The listing builds one solid part. Answer for the finished solid, in the listing's coordinates (mm). A direction names the side the tool comes from. Give positions to 0.01 mm unless a question says otherwise; leave off trailing zeros. Order: outer loops, then holes, each group sorted by start corner. A loop starts at its lowest first (then second) coordinate and runs counter-clockwise, first axis right, second up. Notation, with made-up numbers: (-39.5, 27) - (4.5, 27) arc R14 ccw to (4.5, 43) - close; hole circle Ø11 at (56, 70.25). An arc over 180 degrees is marked (long way). Answer as CSV lines item,"result". Start each with the question number.
1. Flat-ended cylindrical pins translate along their axes: pin 1 (8 mm diameter, centred on x = 14.5, z = -11.5, fed in from -Y); pin 2 (15 mm diameter, centred on x = 9.5, z = -4.5, fed in from -Y); pin 3 (1 mm diameter, centred on y = 0.5, z = 1, fed in from +X). Find the tip coordinate at first contact, or state that the pin passes through.
2. Which of the six approach directions +Z, -Z, +X, -X, +Y, -Y give full straight-line access (tool end or side, diameter ignored) to faces 4 (the cylindrical face through (12.285, 0.986, 9.699)), 5 (the cylindrical face through (-19.976, -0.246, -11.783)), 6 (the flat face through (22, 1, 13))?
3. Consider line 1 along X through (y, z) = (1.5, -10); line 2 along Z through (x, y) = (20, 0.95); line 3 along X through (y, z) = (1.2, 0.25). Determine where each line is inside the solid, lowest interval first. Write a range as [from, to].
4. Determine the mould class of faces 1 (the flat face through (0, 1, 15)), 2 (the flat face through (10, -2.4, -3)), 3 (the flat face through (17, 1, -5)) for opening direction Z: +Z half, -Z half, draft (parallel to the pull), parting line (faces both ways), or undercut.
5. Section C-C on y = 1.05 is taken. Give the vertices of the cut face in (x, z), and give its area (3 significant figures).
6. Section D-D on z = -10 is taken. Give the vertices of the cut face in (x, y).
7. Section B-B on z = 8.5 is taken. Give the vertices of the cut face in (x, y), and give its area (3 significant figures).
8. Section A-A on x = 17 is taken. Give the vertices of the cut face in (y, z), and give its area (3 significant figures).
from build123d import *

# Parameters (mm, degrees)
SKETCH1_W           = 44
SKETCH1_H           = 30
SKETCH1_R           = 1.2192
SKETCH1_R_2         = 1.55
BOSS_EXTRUDE1_DEPTH = 2
SKETCH2_R           = 1
BOSS_EXTRUDE2_DEPTH = 1.5
FILLET1_R           = 1
SKETCH4_R           = 1
BOSS_EXTRUDE3_DEPTH = 2.4
SKETCH5_W           = 10
SKETCH5_H           = 15
CUT_EXTRUDE1_DEPTH  = 27.988145546
FILLET2_R           = 1


with BuildPart() as part:
    # Sketch1 → Boss-Extrude1 (new body)
    with BuildSketch(Plane(origin=(0, 0, 0), x_dir=(1, 0, 0), z_dir=(0, 1, 0))):
        Rectangle(SKETCH1_W, SKETCH1_H)
        with Locations(Location((17, 10, 0), (0, 0, 270))):
            Circle(SKETCH1_R, mode=Mode.SUBTRACT)
        with Locations(Location((-6, 10, 0), (0, 0, 270))):
            Circle(SKETCH1_R_2, mode=Mode.SUBTRACT)
    extrude(amount=BOSS_EXTRUDE1_DEPTH)

    # Sketch2 → Boss-Extrude2 (add)
    with BuildSketch(Plane(origin=(0, 0, 0), x_dir=(-1, 0, 0), z_dir=(0, -1, 0))):
        with Locations(Location((19, 12, 0), (0, 0, 90))):
            Circle(SKETCH2_R)
        with Locations(Location((-10, -12.5, 0), (0, 0, 90))):
            Circle(SKETCH2_R)
    extrude(amount=BOSS_EXTRUDE2_DEPTH)

    # Fillet1
    fillet1_edges = [part.edges().sort_by_distance(p)[0] for p in [
        (-19, -1.5, -11),
        (10, -1.5, 13.5),
    ]]
    fillet(fillet1_edges, radius=FILLET1_R)

    # Sketch4 → Boss-Extrude3 (add)
    with BuildSketch(Plane.XZ):
        with Locations(Location((10, 8.5, 0), (0, 0, 270))):
            Circle(SKETCH4_R)
        with Locations(Location((-18.5, -3.5, 0), (0, 0, 270))):
            Circle(SKETCH4_R)
        with Locations(Location((10, -3.5, 0), (0, 0, 270))):
            Circle(SKETCH4_R)
    extrude(amount=BOSS_EXTRUDE3_DEPTH)

    # Sketch5 → Cut-Extrude1 (cut, through all)
    with BuildSketch(Plane(origin=(0, 2, 0), x_dir=(1, 0, 0), z_dir=(0, 1, 0))):
        with Locations((17, -2.5)):
            Rectangle(SKETCH5_W, SKETCH5_H)
    extrude(amount=-CUT_EXTRUDE1_DEPTH, mode=Mode.SUBTRACT)

    # Fillet2
    fillet2_edges = [part.edges().sort_by_distance(p)[0] for p in [
        (12, 1, 10),
        (12, 1, -5),
    ]]
    fillet(fillet2_edges, radius=FILLET2_R)


solid = part.part
Checks:
1,pin 1,"stops at y = 0"
1,pin 2,"stops at y = -2.4"
1,pin 3,"stops at x = 12"
2,face 4,"+X, +Y, -Y"
2,face 5,"-Y"
2,face 6,"+Z, -Z, +X, +Y, -Y"
3,line 1,"x = [-22, -7.55], [-4.45, 15.78], [18.22, 22]"
3,line 2,"z = [-15, -5], [10, 15]"
3,line 3,"x = [-22, 12]"
4,face 1,"+Z half"
4,face 2,"draft"
4,face 3,"undercut"
5,outline,"(-22, -15) - (22, -15) - (22, -5) - (13, -5) arc R1 cw to (12, -4) - (12, 9) arc R1 cw to (13, 10) - (22, 10) - (22, 15) - (-22, 15) - close; hole circle Ø3.1 at (-6, -10); hole circle Ø2.44 at (17, -10)"
5,area,"1,160 mm²"
6,outline,"(-22, 0) - (-7.55, 0) - (-7.55, 2) - (-22, 2) - close; (-4.45, 0) - (15.78, 0) - (15.78, 2) - (-4.45, 2) - close; (18.22, 0) - (22, 0) - (22, 2) - (18.22, 2) - close"
7,outline,"(-22, 0) - (9, 0) - (9, -2.4) - (11, -2.4) - (11, 0) - (12, 0) - (12, 2) - (-22, 2) - close"
7,area,"72.8 mm²"
8,outline,"(0, -15) - (2, -15) - (2, -11.22) - (0, -11.22) - close; (0, -8.78) - (2, -8.78) - (2, -5) - (0, -5) - close; (0, 10) - (2, 10) - (2, 15) - (0, 15) - close"
8,area,"25.1 mm²"
